```python
from build123d import *

# Parameters (mm, degrees)
SKETCH1_W               = 48.1584
SKETCH1_H               = 36.068
SKETCH1_R               = 9.525
BASE_FLANGE1_DEPTH      = 1.27
EDGE_FLANGE1_DEPTH      = 48.1584
EDGE_FLANGE1_START      = 1.27
EDGE_FLANGE1_PROFILE_W  = 48.1584
EDGE_FLANGE1_PROFILE_H  = 19.7612
EDGE_FLANGE1_PROFILE_R  = 4.73075
EDGE_FLANGE1_FLAT_DEPTH = 1.27
CUT_EXTRUDE7_DEPTH      = 53.108321313
FILLET2_R               = 7.62
FILLET3_R               = 3.81


# Sheet-metal steps are written as plain solids
with BuildPart() as part:
    # Sketch1 → Base-Flange1 (new body)
    with BuildSketch(Plane(origin=(0, 0, 0), x_dir=(1, 0, 0), z_dir=(0, 1, 0))):
        Rectangle(SKETCH1_W, SKETCH1_H)
        with Locations(Location((0, 0, 0), (0, 0, 270))):
            Circle(SKETCH1_R, mode=Mode.SUBTRACT)
    extrude(amount=-BASE_FLANGE1_DEPTH)

    # Edge-Flange1 bend section (across the edge) → Edge-Flange1 (add)
    with BuildSketch(Plane(origin=(24.0792, 0, -19.304), x_dir=(0, 0, 1), z_dir=(-1, 0, 0))):
        with BuildLine():
            Line((-1.27, 1.27), (0, 1.27))
            ThreePointArc((0, 1.27), (0.371974388, 0.371974388), (1.27, 0))
            Line((1.27, 0), (1.27, -1.27))
            ThreePointArc((1.27, -1.27), (-0.526051224, -0.526051224), (-1.27, 1.27))
        make_face()
    edge_flange1 = extrude(amount=EDGE_FLANGE1_DEPTH)

    # Edge-Flange1 profile (on flange) → Edge-Flange1 flat (add)
    with BuildSketch(Plane(origin=(0, 0, -19.304), x_dir=(-1, 0, 0), z_dir=(0, 0, -1)).offset(EDGE_FLANGE1_START)):
        with Locations((0, 11.1506)):
            Rectangle(EDGE_FLANGE1_PROFILE_W, EDGE_FLANGE1_PROFILE_H)
        with Locations((-15.113, 12.065)):
            Circle(EDGE_FLANGE1_PROFILE_R, mode=Mode.SUBTRACT)
        with Locations((15.113, 12.065)):
            Circle(EDGE_FLANGE1_PROFILE_R, mode=Mode.SUBTRACT)
    edge_flange1_flat = extrude(amount=-EDGE_FLANGE1_FLAT_DEPTH)

    # Mirror1: Edge-Flange1, Edge-Flange1 flat across plane
    add(edge_flange1.mirror(Plane.XY))
    add(edge_flange1_flat.mirror(Plane.XY))

    # Sketch11 → Cut-Extrude7 (cut, through all)
    with BuildSketch(Plane(origin=(0, 0, -20.574), x_dir=(-1, 0, 0), z_dir=(0, 0, -1))):
        with BuildLine():
            Line((24.0792, 19.431), (24.0792, 21.0312))
            Line((24.0792, 21.0312), (-24.0792, 21.0312))
            Line((-24.0792, 21.0312), (-24.0792, 19.431))
            Line((-24.0792, 19.431), (-15.113, 19.431))
            ThreePointArc((-15.113, 19.431), (-9.90445145, 17.27354855), (-7.747, 12.065))
            Line((-7.747, 12.065), (7.747, 12.065))
            ThreePointArc((7.747, 12.065), (9.90445145, 17.27354855), (15.113, 19.431))
            Line((15.113, 19.431), (24.0792, 19.431))
        make_face()
    extrude(amount=-CUT_EXTRUDE7_DEPTH, mode=Mode.SUBTRACT)

    # Fillet2
    fillet2_edges = [part.edges().sort_by_distance(p)[0] for p in [
        (7.747, 12.065, -19.939),
        (-7.747, 12.065, -19.939),
        (7.747, 12.065, 19.939),
        (-7.747, 12.065, 19.939),
    ]]
    fillet(fillet2_edges, radius=FILLET2_R)

    # Fillet3
    fillet3_edges = [part.edges().sort_by_distance(p)[0] for p in [
        (-24.0792, 19.431, -19.939),
        (24.0792, 19.431, -19.939),
        (24.0792, 19.431, 19.939),
        (-24.0792, 19.431, 19.939),
    ]]
    fillet(fillet3_edges, radius=FILLET3_R)


solid = part.part
```
The model under review builds one solid part; all positions refer to its coordinate system, in mm. A direction names the side the tool comes from. Give positions to 0.01 mm unless a question says otherwise; leave off trailing zeros. Write each loop counter-clockwise with the first axis right and the second up, starting at its lowest first coordinate (ties: lowest second). Pieces come first, ordered by that corner, then holes.
(1) Consider section A-A, the plane y = 6.5. Give the boundary of the cut face in (x, z), and give its area (3 significant figures).
(2) The part is to be moulded in two halves that separate along Z. For faces 1 (the cylindrical face through (0.337, -0.546, 19.81)), 2 (the flat face through (0, 12.065, -20)), 3 (the cylindrical face through (0.34, 0.38, 18.94)), say which applies: released by +Z, released by -Z, zero draft, split by the parting line, or undercut.
(3) Tool access review of faces 4 (the cylindrical face through (-22.99, 18.29, 19.95)), 5 (the cylindrical face through (6.03, 13.09, -19.93)), 6 (the flat face through (0, 8, 19.304)): name each direction out of +Z, -Z, +X, -X, +Y, -Y from which nothing blocks a thin tool from reaching the whole face with its end or side.
(4) To check wall thickness, follow L1, parallel to Z at x = -1, y = 2; L2, parallel to X at y = -0.95, z = 0 (3 decimals); L3, parallel to Y at x = 10, z = 17. State the ranges of each line that lie inside material, in increasing order.
(5) Consider section D-D, the plane y = 10.75. Give the boundary of the cut face in (x, z), and give its area (3 significant figures).
(6) Consider section B-B, the plane x = 0. Give the boundary of the cut face in (y, z) (3 decimals).
(7) For P1, Ø1.5, axis at x = 13.5, z = 13.5, coming from the +Y side, flat-tipped, find the tip position at first contact; note if it passes through.
(8) Consider section C-C, the plane z = 0. Give the boundary of the cut face in (x, y) (3 decimals).
Returned:
1. outline: (-24.08, -20.57) - (24.08, -20.57) - (24.08, -19.3) - (-24.08, -19.3) - close; (-24.08, 19.3) - (24.08, 19.3) - (24.08, 20.57) - (-24.08, 20.57) - close
1. area: 122 mm2
2. face 1: released by +Z
2. face 2: zero draft
2. face 3: undercut
3. face 4: +Z, -Z, -X, +Y
3. face 5: +Z, -Z, +Y
3. face 6: +X, -X, +Y
4. L1: z = -20.57 to -19.3, 19.3 to 20.57
4. L2: x = -24.079 to -9.525, 9.525 to 24.079
4. L3: y = -1.27 to 0
5. outline: (-24.08, -20.57) - (-19.66, -20.57) - (-19.66, -19.3) - (-24.08, -19.3) - close; (-24.08, 19.3) - (-19.66, 19.3) - (-19.66, 20.57) - (-24.08, 20.57) - close; (-10.57, -20.57) - (10.57, -20.57) - (10.57, -19.3) - (-10.57, -19.3) - close; (-10.57, 19.3) - (10.57, 19.3) - (10.57, 20.57) - (-10.57, 20.57) - close; (19.66, -20.57) - (24.08, -20.57) - (24.08, -19.3) - (19.66, -19.3) - close; (19.66, 19.3) - (24.08, 19.3) - (24.08, 20.57) - (19.66, 20.57) - close
5. area: 76.2 mm2
6. outline: (-1.27, -18.034) arc R2.54 ccw to (1.27, -20.574) - (12.065, -20.574) - (12.065, -19.304) - (1.27, -19.304) arc R1.27 cw to (0, -18.034) - (0, -9.525) - (-1.27, -9.525) - close; (-1.27, 9.525) - (0, 9.525) - (0, 18.034) arc R1.27 cw to (1.27, 19.304) - (12.065, 19.304) - (12.065, 20.574) - (1.27, 20.574) arc R2.54 ccw to (-1.27, 18.034) - close
7. P1: stops at y = 0
8. outline: (-24.079, -1.27) - (-9.525, -1.27) - (-9.525, 0) - (-24.079, 0) - close; (9.525, -1.27) - (24.079, -1.27) - (24.079, 0) - (9.525, 0) - close
